Can you work these out from the model? Positions are in its coordinate system, mm. Face numbers are marked on the shaded views. A direction names the side the tool comes from. Give positions to 0.01 mm unless a question says otherwise; leave off trailing zeros. Order: outer loops, then holes, each group sorted by start corner. A loop starts at its lowest first (then second) coordinate and runs counter-clockwise, first axis right, second up. Notation, with made-up numbers: M 52.5,-27 L 102.5,-27 A25 ccw 102.5,7 Z; hole C 30.5,-27 d4. An arc over 180 degrees is marked long. Answer as a JSON object with one key per item and string values.
```python
from build123d import *

# Parameters (mm, degrees)
SKETCH_R     = 7.5
PAD_DEPTH    = 30
SKETCH001_R  = 1.7
POCKET_DEPTH = 61.001
FILLET_R     = 0.5


with BuildPart() as part:
    # Sketch → Pad (new body)
    with BuildSketch(Plane.XY):
        Polygon((7.5, -11), (17, -11), (17, -6), (15.5, -3.5), (15.5, 6), (8.5, 6), (5, 11), (0, 11), (-5, 11), (-8.5, 6), (-15.5, 6), (-15.5, -3.5), (-17, -6), (-17, -11), (-7.5, -11), (-6, -10), (0, -10), (6, -10), align=None)
        Circle(SKETCH_R, mode=Mode.SUBTRACT)
    extrude(amount=PAD_DEPTH)

    # Sketch001 → Pocket (cut, through all)
    with BuildSketch(Plane.XZ.offset(-50)):
        with Locations((-12, 24)):
            Circle(SKETCH001_R)
        with Locations((12, 24)):
            Circle(SKETCH001_R)
        with Locations((-12, 6)):
            Circle(SKETCH001_R)
        with Locations((12, 6)):
            Circle(SKETCH001_R)
    extrude(amount=POCKET_DEPTH, mode=Mode.SUBTRACT)

    # Fillet
    fillet_edges = [part.edges().sort_by_distance(p)[0] for p in [
        (-5, 11, 15),
        (5, 11, 15),
        (-15.5, 6, 15),
        (-17, -6, 15),
        (15.5, 6, 15),
        (17, -6, 15),
        (-7.5, -11, 15),
        (7.5, -11, 15),
        (-8.5, 6, 15),
        (8.5, 6, 15),
        (-15.5, -3.5, 15),
        (15.5, -3.5, 15),
    ]]
    fillet(fillet_edges, radius=FILLET_R)


solid = part.part
```
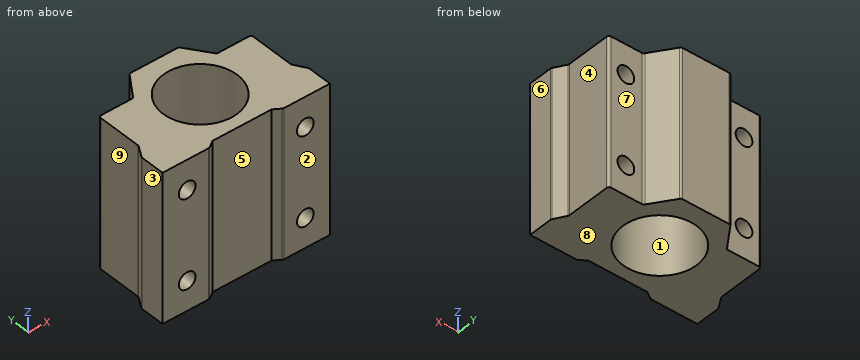
1) I want a section at D-D on z = 6. Count the separate pieces of the cut face and the enclosed holes in it, and give its area (3 significant figures).
Results found:
{"separate pieces": "3", "enclosed holes": "1", "area": "307 mm²"}
2) I want a section at B-B on x = 12. Write out the boundary of the cut face in (y, z).
Results found:
{"outline": "M -11,0 L 6,0 L 6,4.3 L -11,4.3 Z; M -11,7.7 L 6,7.7 L 6,22.3 L -11,22.3 Z; M -11,25.7 L 6,25.7 L 6,30 L -11,30 Z"}
3) I want a section at A-A on y = 0. Write out the boundary of the cut face in (x, z), and give its area (3 significant figures).
Results found:
{"outline": "M -15.5,0 L -7.5,0 L -7.5,30 L -15.5,30 Z; M 7.5,0 L 15.5,0 L 15.5,30 L 7.5,30 Z; hole C -12,6 d3.4; hole C -12,24 d3.4; hole C 12,6 d3.4; hole C 12,24 d3.4", "area": "444 mm²"}
4) For the marked faces 5, 6, 7, 8 and 9, which set-ups out of +Z, -Z, +X, -X, +Y, -Y let a thin tool reach every point of the face, with its end or its side?
Results found:
{"face 5": "+Z, -Z, -Y", "face 6": "+Z, -Z, +X, +Y, -Y", "face 7": "+Z, -Z, +X, +Y", "face 8": "-Z, +X, -X, +Y, -Y", "face 9": "+Z, -Z, -X, +Y"}
5) I'm going to push flat-ended pins straight in: pin 1 Ø4.5 at (y, z) = (0.5, 14.5) entering from -X; pin 2 Ø5.5 at (x, z) = (12, 24) entering from +Y; pin 3 Ø4 at (y, z) = (1.5, 7) entering from +X; pin 4 Ø2 at (x, z) = (-12, 24) entering from -Y. Where does each tip first touch, or does it pass through?
Results found:
{"pin 1": "stops at x = -15.5", "pin 2": "stops at y = 6", "pin 3": "stops at x = 15.5", "pin 4": "passes through"}
6) I want a section at C-C on x = 0. Write out the boundary of the cut face in (y, z).
Results found:
{"outline": "M -10,0 L -7.5,0 L -7.5,30 L -10,30 Z; M 7.5,0 L 11,0 L 11,30 L 7.5,30 Z"}
7) I need wall thicknesses on L1, parallel to Z at x = -12, y = -4.75; L2, parallel to X at y = -4.5, z = 24; L3, parallel to Z at x = -13, y = -8.5. Which ranges of each line are inside material? Lowest first, please.
Results found:
{"L1": "z = 0 to 4.3, 7.7 to 22.3, 25.7 to 30", "L2": "x = -16.1 to -13.7, -10.3 to -6, 6 to 10.3, 13.7 to 16.1", "L3": "z = 0 to 4.63, 7.37 to 22.63, 25.37 to 30"}
8) Thinking about a two-plate mould opening in X: for the marked faces 1, 2, 3 and 4, which applies, pulls with the +X half, pulls with the -X half, needs draft (parallel to the pull), parting line crosses it, or undercut?
Results found:
{"face 1": "undercut", "face 2": "needs draft", "face 3": "pulls with the -X half", "face 4": "pulls with the +X half"}
